The model under review builds one solid part; all positions refer to its coordinate system, in mm. Face numbers are marked on the shaded views. A direction names the side the tool comes from. Give positions to 0.01 mm unless a question says otherwise; leave off trailing zeros. Order: outer loops, then holes, each group sorted by start corner. A loop starts at its lowest first (then second) coordinate and runs counter-clockwise, first axis right, second up. Notation, with made-up numbers: (-20, -28.5) - (30, -28.5) arc R9 ccw to (30, -21.5) - close; hole circle Ø3 at (36, 55.25). An arc over 180 degrees is marked (long way). Write item = value, one per line. Start each with the question number.
1. Wall thickness on probe 1 along Z at (x, y) = (1, -2.25); probe 2 along Y at (x, z) = (-0.5, -2.6); probe 3 along X at (y, z) = (-1, -0.85): over which ranges is each line inside the solid? List them lowest first.
2. Machinability: for the marked faces 1, 2, 3, 4 and 5, which of the approach directions +Z, -Z, +X, -X, +Y, -Y give a long, thin tool a straight path to every point of the face, cutting with its end or side? Answer none if there is none.
3. We need section A-A, the plane x = 0. Give the boundary of the cut face in (y, z), and give its area (3 significant figures).
4. For P1, Ø1.2, axis at x = 0, z = -1, coming from the -Y side; P2, Ø1.5, axis at x = 0.5, y = 3, coming from the -Z side; P3, Ø1.5, axis at x = -1.5, z = -1, coming from the +Y side, all flat-tipped, find the tip position at first contact; note any pin that passes through.
5. We need section B-B, the plane z = -2.25. Give the boundary of the cut face in (x, y), and give its area (3 significant figures).
from build123d import *

# Parameters (mm, degrees)
F0_R     = 6
F1_DEPTH = 0.5
F3_DEPTH = 3
F4_R     = 0.5
F5_R     = 0.25


with BuildPart() as f1:
    # F0 (on Top) → F1 (new body)
    with BuildSketch(Plane.XY):
        Circle(F0_R)
    extrude(amount=F1_DEPTH)

    # F2 (on face) → F3 (join)
    with BuildSketch(Plane(origin=(0, 0, 0), x_dir=(1, 0, 0), z_dir=(0, 0, -1))):
        Polygon((-1.154701, -2), (1.154701, -2), (2.309401, 0), (1.154701, 2), (-1.154701, 2), (-2.309401, 0), align=None)
    extrude(amount=F3_DEPTH)

    # F4
    f4_edges = [f1.edges().sort_by_distance(p)[0] for p in [
        (-1.732051, 1, -3),
        (0, 2, -3),
        (1.732051, 1, -3),
        (1.732051, -1, -3),
        (0, -2, -3),
        (-1.732051, -1, -3),
    ]]
    fillet(f4_edges, radius=F4_R)

    # F5
    f5_edges = [f1.edges().sort_by_distance(p)[0] for p in [
        (-6, 0, 0.5),
    ]]
    fillet(f5_edges, radius=F5_R)


solid = f1.part
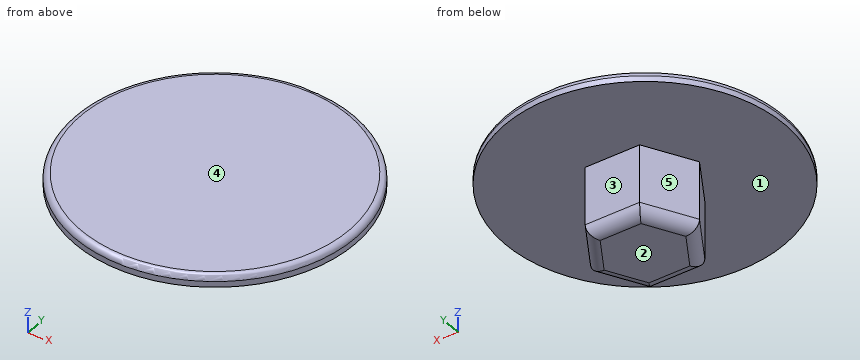
Model answer:
q1.probe_1 = 0 to 0.5
q1.probe_2 = -1.99 to 1.99
q1.probe_3 = -1.73 to 1.73
q2.face_1 = -Z
q2.face_2 = -Z, +X, -X, +Y, -Y
q2.face_3 = -Z, +X, -X, +Y
q2.face_4 = +Z, +X, -X, +Y, -Y
q2.face_5 = -Z, -X, +Y
q3.outline = (-6, 0) - (-2, 0) - (-2, -2.5) arc R0.5 ccw to (-1.5, -3) - (1.5, -3) arc R0.5 ccw to (2, -2.5) - (2, 0) - (6, 0) - (6, 0.25) arc R0.25 ccw to (5.75, 0.5) - (-5.75, 0.5) arc R0.25 ccw to (-6, 0.25) - close
q3.area = 17.9 mm2
q4.P1 = -2
q4.P2 = 0
q4.P3 = 2
q5.outline = (-2.31, 0) - (-1.15, -2) - (1.15, -2) - (2.31, 0) - (1.15, 2) - (-1.15, 2) - close
q5.area = 13.9 mm2
